Read the model definition and answer for the solid it produces. Units are mm, in the model's axes. A direction names the side the tool comes from. Give positions to 0.01 mm unless a question says otherwise; leave off trailing zeros. Loops run counter-clockwise (first coordinate to the right, second up) from the corner with the lowest first, then second, coordinate; pieces in that order, holes last. Notation, with made-up numbers: (-9.75, -8) - (6.25, -8) arc R26 cw to (6.25, 13) - close; hole circle Ø11 at (61.5, 47). An arc over 180 degrees is marked (long way). Write item = value, one per line.
Autodesk Inventor part; units mm, degrees
ref_plane "YZ Plane" through (0, 0, 0) normal (1, 0, 0) x (0, 1, 0)
ref_plane "XZ Plane" through (0, 0, 0) normal (0, 1, 0) x (-1, 0, 0)
ref_plane "XY Plane" through (0, 0, 0) normal (0, 0, 1) x (1, 0, 0)
sketch "Sketch1" plane through (0, 0, 0) normal (0, 1, 0) x (-1, 0, 0)
  circle A0 centre (0, 0) radius 5
  circle A1 centre (0, 0) radius 4
  dimension "d0" = 10
  dimension "d1" = 8
extrude "Extrusion1" add sketch "Sketch1" along normal blind 60
sketch "Sketch2" plane through (0, 0, 0) normal (1, 0, 0) x (0, 1, 0)
  circle A0 centre (55, 0) radius 5
  line L0 (60, 4) -> (60, -4)
  circle A1 centre (55, 0) radius 1
  line L1 (55, -5) -> (60, -5)
  line L2 (0, -5) -> (60, -5)
  line L3 (60, -5) -> (60, 5)
  line L4 (55, 5) -> (60, 5)
  line L5 (60, 5) -> (60, -5)
  point P0 (0, 0)
  point P1 (60, 0)
  point P2 (60, 0)
  dimension "d4" = 10
  dimension "d5" = 5
  dimension "d6" = 0
  dimension "d7" = 2
extrude "Extrusion2" cut sketch "Sketch2" along normal through all both and the other way through all contours L0 L3 L1 A0 | A0 L4 L3 L0 | A1
sketch "Sketch3" plane through (0, 0, 0) normal (0, 0, 1) x (1, 0, 0)
  line L0 (-1.25, 60) -> (1.25, 60)
  line L1 (1.25, 60) -> (1.25, 50)
  line L2 (1.25, 50) -> (-1.25, 50)
  line L3 (-1.25, 50) -> (-1.25, 60)
  line L4 (-5, 0) -> (-5, 60)
  line L5 (5, 60) -> (-5, 60)
  point P0 (0, 0)
  point P1 (0, 50)
  dimension "d10" = 2.5
  dimension "d11" = 10
  dimension "d12" = 0
  dimension "d13" = 5
extrude "Extrusion3" cut sketch "Sketch3" along normal through all both and the other way through all
properties part number "Shaft" material "Stainless Steel"
1) A cutting plane is placed at B-B on z = 0. Determine the outline of the cut face in (x, y), then the cut area to 3 significant figures.
Output:
outline = (-5, 0) - (-4, 0) - (-4, 54) - (-5, 54) - close; (-5, 56) - (-4, 56) - (-4, 60) - (-5, 60) - close; (4, 0) - (5, 0) - (5, 54) - (4, 54) - close; (4, 56) - (5, 56) - (5, 60) - (4, 60) - close
area = 116 mm²
2) The mould has two halves that part along Z. Classify faces 3 (the face through (-4.2, 60, 0)), 4 (the face through (4.429, 55.954, -0.3)), 5 (the face through (-1.25, 54, 4)): pulls with the +Z half, pulls with the -Z half, needs draft (parallel to the pull), parting line crosses it, or undercut.
Output:
face_3 = parting line crosses it
face_4 = undercut
face_5 = needs draft
3) A tool of negligible diameter and unlimited length cuts with its end or side. For faces 1 (the face through (-3.695, 29.581, 1.532)), 2 (the face through (1.25, 54, 4)), from which of +Z, -Z, +X, -X, +Y, -Y can it reach the whole face along a straight path? Write none if from no direction.
Output:
face_1 = +Y, -Y
face_2 = +Z, -Z, +Y
4) Each of these flat-tipped pins is pushed along its axis until it touches: P1, Ø3, axis at x = 2, y = 23, coming from the -Z side; P2, Ø0.8, axis at y = 54, z = 4.5, coming from the +X side; P3, Ø1.1, axis at y = 53.5, z = 4.5, coming from the -X side. Where does it stop, or does it pass through?
Output:
P1 = -4.97
P2 = 2.86
P3 = -3.07
5) A cutting plane is placed at D-D on y = 55. Determine the outline of the cut face in (x, z).
Output:
outline = (-4.9, -1) arc R5 ccw to (-1.25, -4.84) - (-1.25, -3.8) arc R4 cw to (-3.87, -1) - close; (-4.9, 1) - (-3.87, 1) arc R4 cw to (-1.25, 3.8) - (-1.25, 4.84) arc R5 ccw to start; (1.25, -4.84) arc R5 ccw to (4.9, -1) - (3.87, -1) arc R4 cw to (1.25, -3.8) - close; (1.25, 3.8) arc R4 cw to (3.87, 1) - (4.9, 1) arc R5 ccw to (1.25, 4.84) - close
6) Find the intervals of material crossed by probe 1 along X at (y, z) = (29.5, 0); probe 2 along X at (y, z) = (49, 1.25), in increasing order.
Output:
probe_1 = -5 to -4, 4 to 5
probe_2 = -4.84 to -3.8, 3.8 to 4.84
7) A cutting plane is placed at C-C on z = 3. Determine the outline of the cut face in (x, y), then the cut area to 3 significant figures.
Output:
outline = (-4, 0) - (-2.65, 0) - (-2.65, 59) - (-4, 59) - close; (2.65, 0) - (4, 0) - (4, 59) - (2.65, 59) - close
area = 160 mm²
8) A cutting plane is placed at A-A on x = 0. Determine the outline of the cut face in (y, z), then the cut area to 3 significant figures.
Output:
outline = (0, -5) - (50, -5) - (50, -4) - (0, -4) - close; (0, 4) - (50, 4) - (50, 5) - (0, 5) - close
area = 100 mm²
